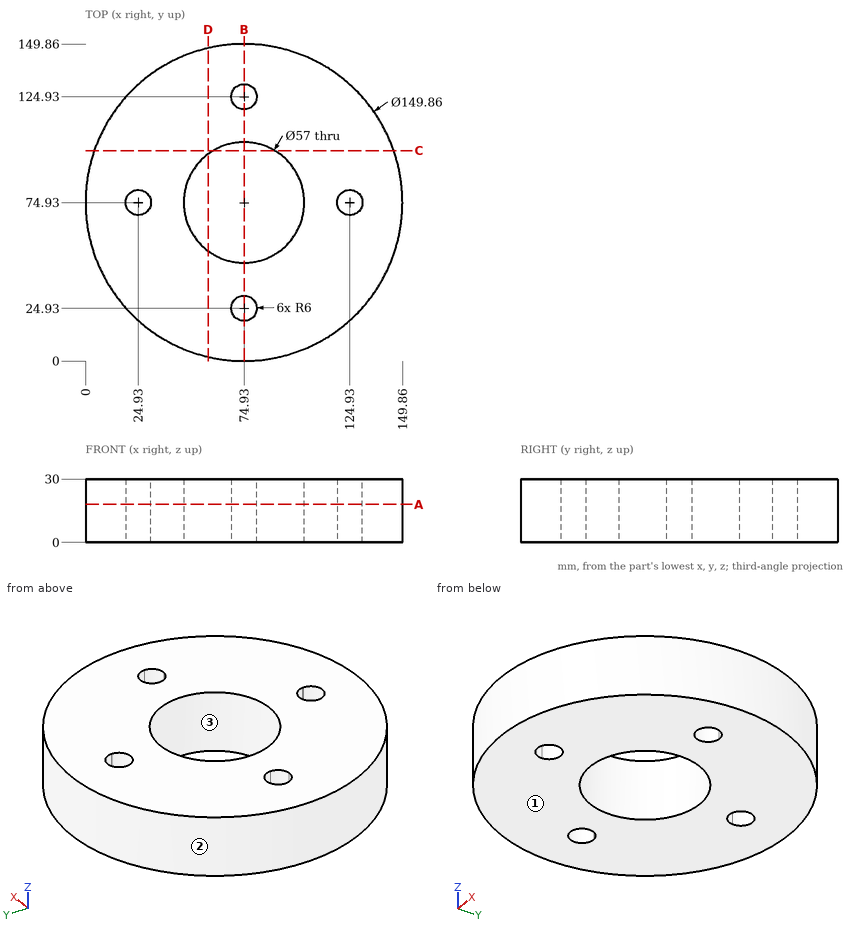
The figure shows three views and two pictorial views of one solid part (mm, origin at its lowest corner). Answer the questions. Give positions to 0.01 mm unless a question says otherwise; leave off trailing zeros. Loops run counter-clockwise (first coordinate to the right, second up) from the corner with the lowest first, then second, coordinate; pieces in that order, holes last. Notation, with made-up numbers: (88, 75) - (108, 75) arc R25 ccw to (108, 93) - close; hole circle Ø7 at (-29.5, 74.5). An arc over 180 degrees is marked (long way). Use one line per item in the form item = value.
1. Section D-D on x = 58 is taken. Give the vertices of the cut face in (y, z), then the cut area to 3 significant figures.
Calculated:
outline = (1.94, 0) - (52, 0) - (52, 30) - (1.94, 30) - close; (97.86, 0) - (147.92, 0) - (147.92, 30) - (97.86, 30) - close
area = 3,000 mm^2
2. The mould has two halves that part along X. Classify the marked faces 1, 2 and 3: pulls with the +X half, pulls with the -X half, needs draft (parallel to the pull), parting line crosses it, or undercut.
Calculated:
face_1 = needs draft
face_2 = parting line crosses it
face_3 = undercut
3. Section A-A on z = 18 is taken. Give the vertices of the cut face in (x, y), then the cut area to 3 significant figures.
Calculated:
outline = circle Ø149.86 at (74.93, 74.93); hole (25.29, 68.94) arc R6 ccw to (30.93, 74.93) arc R6 ccw to (25.29, 80.92) arc R6 ccw (long way) to start; hole circle Ø57 at (74.93, 74.93); hole (80.92, 25.29) arc R6 ccw (long way) to (80.93, 24.93) arc R6 ccw to start; hole (80.92, 124.57) arc R6 ccw to (80.93, 124.93) arc R6 ccw (long way) to start; hole (124.57, 68.94) arc R6 ccw to (130.93, 74.93) arc R6 ccw to (124.57, 80.92) arc R6 ccw to start
area = 14,600 mm^2
4. Section B-B on x = 74.93 is taken. Give the vertices of the cut face in (y, z).
Calculated:
outline = (0, 0) - (18.93, 0) - (18.93, 30) - (0, 30) - close; (30.93, 0) - (46.43, 0) - (46.43, 30) - (30.93, 30) - close; (103.43, 0) - (118.93, 0) - (118.93, 30) - (103.43, 30) - close; (130.93, 0) - (149.86, 0) - (149.86, 30) - (130.93, 30) - close
5. Section C-C on y = 99.5 is taken. Give the vertices of the cut face in (x, z), then the cut area to 3 significant figures.
Calculated:
outline = (4.14, 0) - (60.49, 0) - (60.49, 30) - (4.14, 30) - close; (89.37, 0) - (145.72, 0) - (145.72, 30) - (89.37, 30) - close
area = 3,380 mm^2
6. Given pin 1 Ø1 at (y, z) = (95.5, 23) entering from -X; pin 2 Ø2 at (y, z) = (44, 5) entering from -X; pin 3 Ø3 at (x, z) = (29, 7.5) entering from -Y; pin 4 Ø1.5 at (x, y) = (97.5, 25.5) entering from -Z, each flat-ended and moving along its own axis, determine where each tip first touches the part or whether it passes through.
Calculated:
pin_1 = 2.74
pin_2 = 6.24
pin_3 = 14.59
pin_4 = 0
7. Find the intervals of material crossed by line 1 along Y through (x, z) = (74.93, 19); line 2 along Y through (x, z) = (76, 27); line 3 along X through (y, z) = (78.5, 28) (1 decimal), in increasing order. Write a range as [from, to].
Calculated:
line_1 = [0, 18.93], [30.93, 46.43], [103.43, 118.93], [130.93, 149.86]
line_2 = [0.01, 19.03], [30.83, 46.45], [103.41, 119.03], [130.83, 149.85]
line_3 = [0.1, 20.1], [29.8, 46.7], [103.2, 120.1], [129.8, 149.8]
